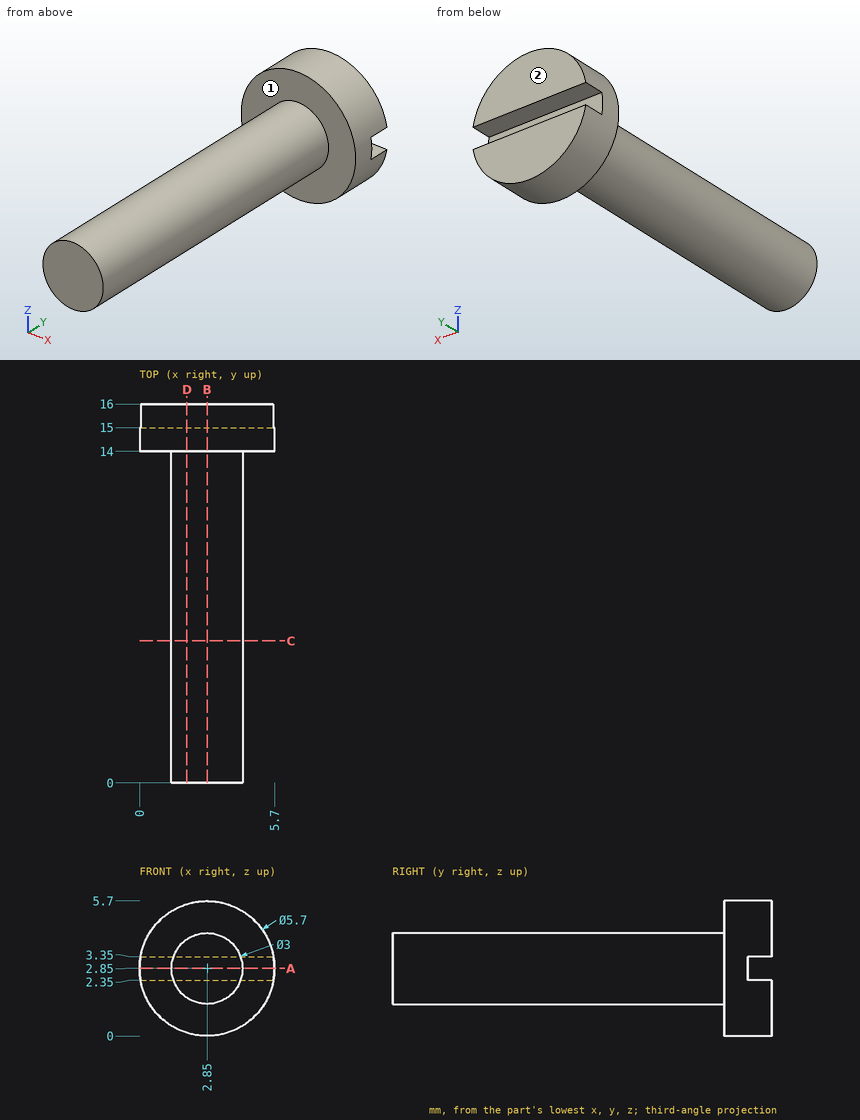
The figure shows three views and two pictorial views of one solid part (mm, origin at its lowest corner). Answer the questions. A direction names the side the tool comes from. Give positions to 0.01 mm unless a question says otherwise; leave off trailing zeros. Write each loop counter-clockwise with the first axis right and the second up, starting at its lowest first coordinate (ties: lowest second). Pieces come first, ordered by that corner, then holes. Notation, with made-up numbers: (-19.5, -33.5) -> (23.5, -33.5) arc R32 ccw to (23.5, -0.5) -> close; hole circle Ø6 at (51, 8.5). An arc over 180 degrees is marked (long way). Answer as a JSON object with one key per item and string values.
1) A tool of negligible diameter and unlimited length cuts with its end or side. For the marked faces 1 and 2, from which of +Z, -Z, +X, -X, +Y, -Y can it reach the whole face along a straight path? Write none if from no direction.
Findings below:
{"face 1": "-Y", "face 2": "+Z, -Z, +X, -X, +Y"}
2) Section D-D on x = 2 is taken. Write down the section's boundary in (y, z).
Findings below:
{"outline": "(0, 1.61) -> (14, 1.61) -> (14, 0.13) -> (16, 0.13) -> (16, 2.35) -> (15, 2.35) -> (15, 3.35) -> (16, 3.35) -> (16, 5.57) -> (14, 5.57) -> (14, 4.09) -> (0, 4.09) -> close"}
3) Section B-B on x = 2.85 is taken. Write down the section's boundary in (y, z), then the cut area to 3 significant figures.
Findings below:
{"outline": "(0, 1.35) -> (14, 1.35) -> (14, 0) -> (16, 0) -> (16, 2.35) -> (15, 2.35) -> (15, 3.35) -> (16, 3.35) -> (16, 5.7) -> (14, 5.7) -> (14, 4.35) -> (0, 4.35) -> close", "area": "52.4 mm^2"}
4) Section C-C on y = 6 is taken. Write down the section's boundary in (x, z), then the cut area to 3 significant figures.
Findings below:
{"outline": "circle Ø3 at (2.85, 2.85)", "area": "7.07 mm^2"}
5) Section A-A on z = 2.85 is taken. Write down the section's boundary in (x, y).
Findings below:
{"outline": "(0, 14) -> (1.35, 14) -> (1.35, 0) -> (4.35, 0) -> (4.35, 14) -> (5.7, 14) -> (5.7, 15) -> (0, 15) -> close"}
6) Flat-ended cylindrical pins translate along their axes: pin 1 Ø1.5 at (x, y) = (2.5, 2) entering from -Z; pin 2 Ø1.5 at (y, z) = (9, 4.5) entering from +X; pin 3 Ø0.8 at (x, z) = (4, 3) entering from +Y; pin 4 Ø0.8 at (x, y) = (4, 15.5) entering from +Z. Find the tip coordinate at first contact, or state that the pin passes through.
Findings below:
{"pin 1": "stops at z = 1.35", "pin 2": "stops at x = 4.05", "pin 3": "stops at y = 16", "pin 4": "stops at z = 5.6"}
7) Straight lines are drawn through the part: probe 1 along Y at (x, z) = (1.6, 4.65); probe 2 along Y at (x, z) = (1.7, 3); probe 3 along X at (y, z) = (11.75, 1.6). For each, find the intervals that lie inside material, in ascending order. Write a range as from..to.
Findings below:
{"probe 1": "y = 14..16", "probe 2": "y = 0..15", "probe 3": "x = 2.02..3.68"}
